Work out the finished part from the listing and answer in its coordinate system (mm). A direction names the side the tool comes from. Round coordinates to 2 decimals unless told otherwise and drop trailing zeros. Loops run counter-clockwise (first coordinate to the right, second up) from the corner with the lowest first, then second, coordinate; pieces in that order, holes last. Notation, with made-up numbers: (49.5, -20.5) -> (95.5, -20.5) arc R29 cw to (95.5, 17.5) -> close; hole circle Ø7 at (8, -35). An arc over 180 degrees is marked (long way). Use one line per item in the form item = value.
```python
from build123d import *

# Parameters (mm, degrees)
SKETCH1_W           = 8
SKETCH1_H           = 66.99
SKETCH1_R           = 1.5
BOSS_EXTRUDE1_DEPTH = 14
FILLET1_R           = 4
SKETCH2_W           = 6
SKETCH2_H           = 10
SKETCH2_H_2         = 11
CUT_EXTRUDE1_DEPTH  = 38.174117676


with BuildPart() as part:
    # Sketch1 → Boss-Extrude1 (new body)
    with BuildSketch(Plane.XY):
        Rectangle(SKETCH1_W, SKETCH1_H)
        with Locations((0, 29.795)):
            Circle(SKETCH1_R, mode=Mode.SUBTRACT)
        with Locations((0, -29.795)):
            Circle(SKETCH1_R, mode=Mode.SUBTRACT)
    extrude(amount=BOSS_EXTRUDE1_DEPTH)

    # Fillet1
    fillet1_edges = [part.edges().sort_by_distance(p)[0] for p in [
        (-4, -33.495, 7),
        (4, -33.495, 7),
        (-4, 33.495, 7),
        (4, 33.495, 7),
    ]]
    fillet(fillet1_edges, radius=FILLET1_R - 0.0001)  # a hair under: the kernel refuses the full size

    # Sketch2 → Cut-Extrude1 (cut, through all)
    with BuildSketch(Plane.ZY.offset(4)):
        with Locations((7, 28.495)):
            Rectangle(SKETCH2_W, SKETCH2_H)
        with Locations((7, -27.995)):
            Rectangle(SKETCH2_W, SKETCH2_H_2)
    extrude(amount=-CUT_EXTRUDE1_DEPTH, mode=Mode.SUBTRACT)


solid = part.part
```
(1) For a pull along Z with two mould halves and no side action, classify faces 4 (the flat face through (0, 0, 0)), 5 (the flat face through (0, -28, 10)), 6 (the flat face through (0, 27, 10)), 7 (the flat face through (-4, 0, 7)) as +Z half, -Z half, draft (parallel to the pull), parting line (faces both ways), or undercut.
Completed:
face_4 = -Z half
face_5 = undercut
face_6 = undercut
face_7 = draft
(2) For faces 1 (the flat face through (4, 0, 7)), 2 (the flat face through (0, -28, 4)), 3 (the flat face through (0, 23.495, 7)), determine the directions among +Z, -Z, +X, -X, +Y, -Y from which every point of the face is accessible in a straight line to the end or side of a thin tool.
Completed:
face_1 = +Z, -Z, +X, +Y, -Y
face_2 = +X, -X, -Y
face_3 = +X, -X, +Y
(3) Given P1, Ø2.5, axis at x = 0, y = -29.795, coming from the +Z side; P2, Ø3, axis at x = -1, z = 6, coming from the +Y side (3 decimals), each flat-ended and moving along its own axis, determine where each tip first touches the part or whether it passes through.
Completed:
P1 = through
P2 = 23.495
(4) Find section B-B, the plane z = 6.75. Write down the section's boundary in (x, y) (3 decimals), then the cut area to 3 significant figures.
Completed:
outline = (-4, -22.495) -> (4, -22.495) -> (4, 23.495) -> (-4, 23.495) -> close
area = 368 mm2
(5) Find section A-A, the plane x = -0.75. Write down the section's boundary in (y, z) (3 decimals), then the cut area to 3 significant figures.
Completed:
outline = (-33.424, 0) -> (-31.094, 0) -> (-31.094, 4) -> (-33.424, 4) -> close; (-33.424, 10) -> (-31.094, 10) -> (-31.094, 14) -> (-33.424, 14) -> close; (-28.496, 0) -> (28.496, 0) -> (28.496, 4) -> (23.495, 4) -> (23.495, 10) -> (28.496, 10) -> (28.496, 14) -> (-28.496, 14) -> (-28.496, 10) -> (-22.495, 10) -> (-22.495, 4) -> (-28.496, 4) -> close; (31.094, 0) -> (33.424, 0) -> (33.424, 4) -> (31.094, 4) -> close; (31.094, 10) -> (33.424, 10) -> (33.424, 14) -> (31.094, 14) -> close
area = 769 mm2
(6) Consider L1, parallel to Y at x = 0, z = 2.7 (3 decimals); L2, parallel to Z at x = -0.75, y = -27.5; L3, parallel to Y at x = -0.5, z = 4.25 (3 decimals). Determine where each line is inside the solid, lowest interval first.
Completed:
L1 = -33.495 to -31.295, -28.295 to 28.295, 31.295 to 33.495
L2 = 0 to 4, 10 to 14
L3 = -22.495 to 23.495
